Can you work these out from the drawing? Everything is in mm from the part's minimum corner. A direction names the side the tool comes from. Coordinates: 2 decimals unless noted, no trailing zeros. Loops run counter-clockwise (first coordinate to the right, second up) from the corner with the lowest first, then second, coordinate; pieces in that order, holes last. Notation, with made-up numbers: (-29, 82.25) -> (-25, 82.25) arc R22 cw to (-25, 110.25) -> close; hole circle Ø7 at (54, 60.5). An arc over 180 degrees is marked (long way). One line per question, with ' | ' between items.
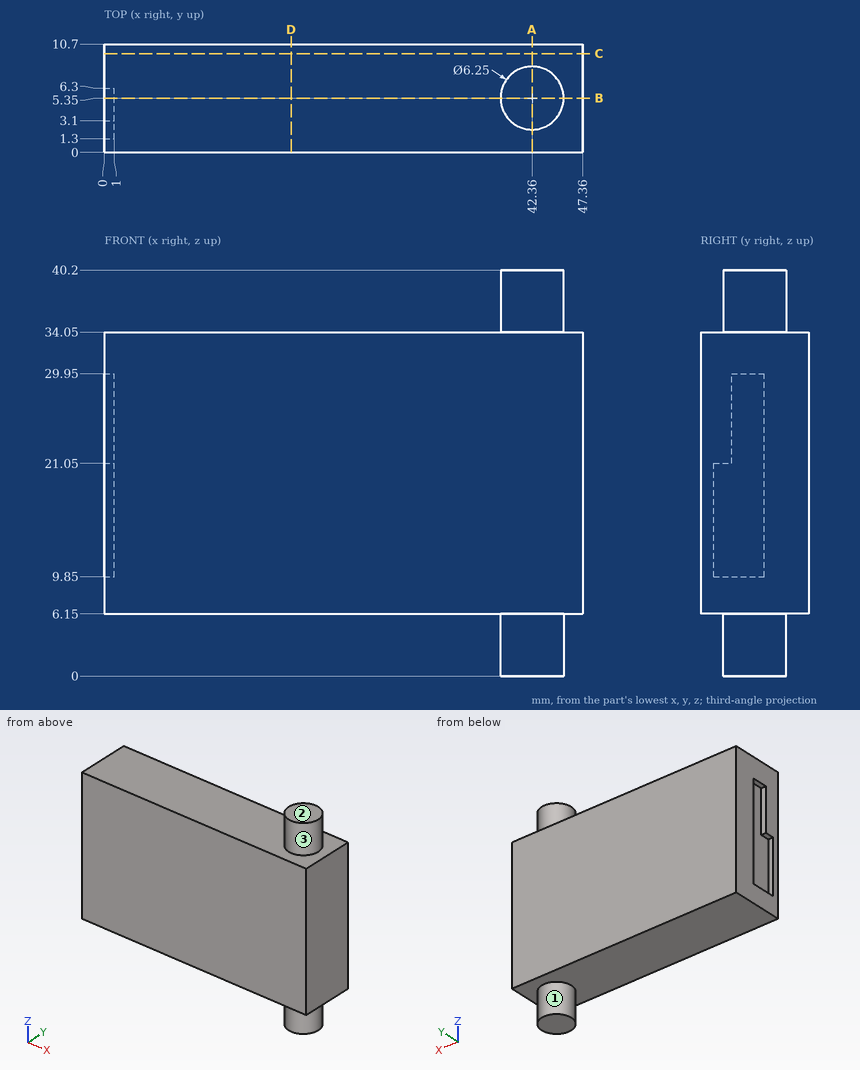
Q1. Imagine slicing it at B-B on y = 5.35. Write out the boundary of the cut face in (x, z) (3 decimals).
Values follow:
outline: (0, 6.15) -> (39.235, 6.15) -> (39.235, 0) -> (45.485, 0) -> (45.485, 6.15) -> (47.36, 6.15) -> (47.36, 34.05) -> (45.485, 34.05) -> (45.485, 40.2) -> (39.235, 40.2) -> (39.235, 34.05) -> (0, 34.05) -> (0, 29.95) -> (1, 29.95) -> (1, 9.85) -> (0, 9.85) -> close
Q2. Imagine slicing it at C-C on y = 9.75. Write out the boundary of the cut face in (x, z).
Values follow:
outline: (0, 6.15) -> (47.36, 6.15) -> (47.36, 34.05) -> (0, 34.05) -> close
Q3. Imagine slicing it at D-D on x = 18.5. Write out the boundary of the cut face in (y, z), plus the area to 3 significant figures.
Values follow:
outline: (0, 6.15) -> (10.7, 6.15) -> (10.7, 34.05) -> (0, 34.05) -> close | area: 299 mm2
Q4. Imagine slicing it at A-A on x = 42.36. Write out the boundary of the cut face in (y, z) (3 decimals).
Values follow:
outline: (0, 6.15) -> (2.225, 6.15) -> (2.225, 0) -> (8.475, 0) -> (8.475, 6.15) -> (10.7, 6.15) -> (10.7, 34.05) -> (8.475, 34.05) -> (8.475, 40.2) -> (2.225, 40.2) -> (2.225, 34.05) -> (0, 34.05) -> close
Q5. For pin 1 (4 mm diameter, centred on y = 4, z = 17, fed in from -X); pin 2 (1.1 mm diameter, centred on x = 0.5, y = 3.5, fed in from +Z); pin 3 (0.8 mm diameter, centred on x = 0.5, y = 2, fed in from -Z), each with a flat end and sliding along its axis, tell me the tip position at first contact or that it passes through.
Values follow:
pin 1: stops at x = 1 | pin 2: stops at z = 34.05 | pin 3: stops at z = 6.15
Q6. Please list where these lines run through material, in increasing order: L1, parallel to Z at x = 37, y = 2.25; L2, parallel to X at y = 4.75, z = 19.5. Write a range as [from, to].
Values follow:
L1: z = [6.15, 34.05] | L2: x = [1, 47.36]
Q7. For the marked faces 1, 2 and 3, which set-ups out of +Z, -Z, +X, -X, +Y, -Y let a thin tool reach every point of the face, with its end or its side?
Values follow:
face 1: -Z | face 2: +Z, +X, -X, +Y, -Y | face 3: +Z
